Source: CAD feature listing. Evaluate the final solid. Frame: model axes, mm. Coordinates: 2 decimals unless noted, no trailing zeros. Write each loop counter-clockwise with the first axis right and the second up, starting at its lowest first coordinate (ties: lowest second). Pieces come first, ordered by that corner, then holes. Notation, with made-up numbers: M 43.5,-39 L 67.5,-39 A36 cw 67.5,-4 Z; hole C 37.5,5 d11. An arc over 180 degrees is marked long. One line per item, written item: value. Start each with the question number.
Item 1: Cut plane B-B, the plane z = -1.1. Output: boundary loops of the cut face in (x, y).
Item 2: Cut plane C-C, the plane x = 34.5. Output: boundary loops of the cut face in (y, z).
Item 3: Cut plane D-D, the plane y = 2.5. Output: boundary loops of the cut face in (x, z).
Item 4: Ray query, L1, parallel to X at y = -0.75, z = 0.9; L2, parallel to X at y = 2.75, z = -0.2; L3, parallel to Y at x = 33, z = 0.7. Return the intervals inside material, ascending. Write a range as from..to.
Item 5: Pin query (flat end, axial travel): P1, Ø1, axis at x = 32.5, y = 3, coming from the +Z side. Return the tip coordinate at first contact, or that it passes through.
Item 6: Cut plane A-A, the plane y = 0. Output: boundary loops of the cut face in (x, z), then the cut area to 3 significant figures.
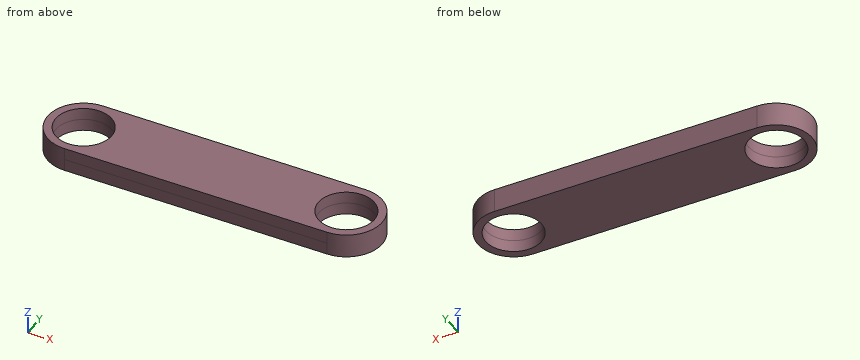
```python
from build123d import *

# Parameters (mm, degrees)
SKETCH_1_R      = 4.5
SKETCH_1_R_2    = 3.5
EXTRUDE_1_DEPTH = 1.5


with BuildPart() as part:
    # Sketch 1 → Extrude 1 (new, symmetric)
    # profile 1 of 3: a face of its own
    with BuildSketch(Plane.XY):
        Circle(SKETCH_1_R)
        Circle(SKETCH_1_R_2, mode=Mode.SUBTRACT)
    # profile 2 of 3: a face of its own
    with BuildSketch(Plane.XY):
        with BuildLine():
            Line((33, 4.5), (0, 4.5))
            ThreePointArc((0, 4.5), (3.181980515, 3.181980515), (4.5, 0))
            ThreePointArc((4.5, 0), (3.181980515, -3.181980515), (0, -4.5))
            Line((0, -4.5), (33, -4.5))
            ThreePointArc((33, -4.5), (28.5, 0), (33, 4.5))
        make_face()
    # profile 3 of 3: a face of its own
    with BuildSketch(Plane.XY):
        with Locations((33, 0)):
            Circle(SKETCH_1_R)
        with Locations((33, 0)):
            Circle(SKETCH_1_R_2, mode=Mode.SUBTRACT)
    extrude(amount=EXTRUDE_1_DEPTH, both=True)


solid = part.part
```
From the geometry:
1. outline: M 0,-4.5 L 33,-4.5 A4.5 ccw 33,4.5 L 0,4.5 A4.5 ccw Z; hole C 0,0 d7; hole C 33,0 d7
2. outline: M -4.24,-1.5 L -3.16,-1.5 L -3.16,1.5 L -4.24,1.5 Z; M 3.16,-1.5 L 4.24,-1.5 L 4.24,1.5 L 3.16,1.5 Z
3. outline: M -3.74,-1.5 L -2.45,-1.5 L -2.45,1.5 L -3.74,1.5 Z; M 2.45,-1.5 L 30.55,-1.5 L 30.55,1.5 L 2.45,1.5 Z; M 35.45,-1.5 L 36.74,-1.5 L 36.74,1.5 L 35.45,1.5 Z
4. L1: x = -4.44..-3.42, 3.42..29.58, 36.42..37.44
4. L2: x = -3.56..-2.17, 2.17..30.83, 35.17..36.56
4. L3: y = -4.5..-3.5, 3.5..4.5
5. P1: stops at z = 1.5
6. outline: M -4.5,-1.5 L -3.5,-1.5 L -3.5,1.5 L -4.5,1.5 Z; M 3.5,-1.5 L 29.5,-1.5 L 29.5,1.5 L 3.5,1.5 Z; M 36.5,-1.5 L 37.5,-1.5 L 37.5,1.5 L 36.5,1.5 Z
6. area: 84.0 mm²
